Design review of the part built by this model. Coordinates are the model's own, in mm. Face numbers are marked on the shaded views. Give positions to 0.01 mm unless a question says otherwise; leave off trailing zeros. Loops run counter-clockwise (first coordinate to the right, second up) from the corner with the lowest first, then second, coordinate; pieces in that order, holes last. Notation, with made-up numbers: M 34.5,65 L 39.5,65 A8 cw 39.5,77 Z; hole C 78.5,33 d10. An arc over 180 degrees is marked long. Answer as CSV lines item,"result".
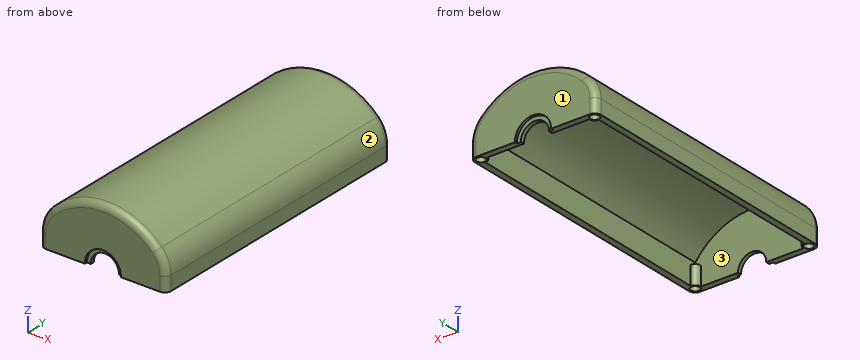
```python
from build123d import *

# Parameters (mm, degrees)
F0_W      = 20
F0_H      = 4
F1_DEPTH  = 45
F2_T      = -1
F3_R      = 5
F4_R      = 5
F6_DEPTH  = 3
F7_R      = 0.7
F8_DEPTH  = 3
F9_R      = 1
F10_R     = 1
F12_DEPTH = 50
F13_DEPTH = 0.4
F15_DEPTH = 0.4


with BuildPart() as f1:
    # F0 (on Front) → F1 (new body)
    with BuildSketch(Plane.XZ):
        with Locations((10, 2)):
            Rectangle(F0_W, F0_H)
        with BuildLine():
            ThreePointArc((20, 4), (10, 9.301808562), (0, 4))
            Line((0, 4), (20, 4))
        make_face()
    extrude(amount=F1_DEPTH)

    # F2
    f2_openings = [f1.faces().sort_by_distance(p)[0] for p in [
        (10, -22.5, 0),
    ]]
    offset(amount=F2_T, openings=f2_openings)

    # F3
    f3_edges = [f1.edges().sort_by_distance(p)[0] for p in [
        (0, -22.5, 4),
    ]]
    fillet(f3_edges, radius=F3_R)

    # F4
    f4_edges = [f1.edges().sort_by_distance(p)[0] for p in [
        (20, -22.5, 4),
    ]]
    fillet(f4_edges, radius=F4_R)

    # F5 (on face) → F6 (join)
    with BuildSketch(Plane(origin=(0, 0, 0), x_dir=(1, 0, 0), z_dir=(0, 0, -1))):
        with BuildLine():
            Line((1, 1), (1.9, 1))
            ThreePointArc((1.9, 1), (1.6363961031, 1.6363961031), (1, 1.9))
            Line((1, 1.9), (1, 1))
        make_face()
        with BuildLine():
            ThreePointArc((19, 1.9), (18.3636038969, 1.6363961031), (18.1, 1))
            Line((18.1, 1), (19, 1))
            Line((19, 1), (19, 1.9))
        make_face()
        with BuildLine():
            ThreePointArc((18.1, 44), (18.3636038969, 43.3636038969), (19, 43.1))
            Line((19, 43.1), (19, 44))
            Line((19, 44), (18.1, 44))
        make_face()
        with BuildLine():
            Line((1, 44), (1, 43.1))
            ThreePointArc((1, 43.1), (1.6363961031, 43.3636038969), (1.9, 44))
            Line((1.9, 44), (1, 44))
        make_face()
    extrude(amount=-F6_DEPTH)

    # F7 (on face) → F8 (cut)
    with BuildSketch(Plane(origin=(0, 0, 0), x_dir=(1, 0, 0), z_dir=(0, 0, -1))):
        with Locations((1, 1)):
            Circle(F7_R)
        with Locations((19, 1)):
            Circle(F7_R)
        with Locations((1, 44)):
            Circle(F7_R)
        with Locations((19, 44)):
            Circle(F7_R)
    extrude(amount=-F8_DEPTH, mode=Mode.SUBTRACT)

    # F9
    f9_edges = [f1.edges().sort_by_distance(p)[0] for p in [
        (20, -45, 1.117556),
        (19.617968, -45, 4.151977),
        (10, -45, 9.301809),
        (0.382032, -45, 4.151977),
        (0, -45, 1.117556),
    ]]
    fillet(f9_edges, radius=F9_R)

    # F10
    f10_edges = [f1.edges().sort_by_distance(p)[0] for p in [
        (0, 0, 1.117556),
        (0.382032, 0, 4.151977),
        (10, 0, 9.301809),
        (19.617968, 0, 4.151977),
        (20, 0, 1.117556),
    ]]
    fillet(f10_edges, radius=F10_R)

    # F11 (on face) → F12 (cut)
    with BuildSketch(Plane.XZ.offset(45)):
        with BuildLine():
            Line((7.7686794017, 0), (12.2313205983, 0))
            ThreePointArc((12.2313205983, 0), (10, 2.2313205983), (7.7686794017, 0))
        make_face()
    extrude(amount=-F12_DEPTH, mode=Mode.SUBTRACT)

    # F11 (on face) → F13 (cut)
    with BuildSketch(Plane.XZ.offset(45)):
        with BuildLine():
            Line((12.2313205983, 0), (12.8707642747, 0))
            ThreePointArc((12.8707642747, 0), (10, 2.8707642747), (7.1292357253, 0))
            Line((7.1292357253, 0), (7.7686794017, 0))
            ThreePointArc((7.7686794017, 0), (10, 2.2313205983), (12.2313205983, 0))
        make_face()
    extrude(amount=-F13_DEPTH, mode=Mode.SUBTRACT)

    # F14 (on face) → F15 (cut)
    with BuildSketch(Plane(origin=(0, 0, 0), x_dir=(-1, 0, 0), z_dir=(0, 1, 0))):
        with BuildLine():
            Line((-7.7686794017, 0), (-7.1292357253, 0))
            ThreePointArc((-7.1292357253, 0), (-10, 2.8707642747), (-12.8707642747, 0))
            Line((-12.8707642747, 0), (-12.2313205983, 0))
            ThreePointArc((-12.2313205983, 0), (-10, 2.2313205983), (-7.7686794017, 0))
        make_face()
    extrude(amount=-F15_DEPTH, mode=Mode.SUBTRACT)


solid = f1.part
```
1. For P1, Ø2, axis at y = -12, z = 5, coming from the -X side; P2, Ø1.3, axis at x = 1, y = -1, coming from the +Z side; P3, Ø3, axis at x = 9, z = 0.5, coming from the +Y side, all flat-tipped, find the tip position at first contact; note any pin that passes through.
Answer block:
P1,"x = 0.32"
P2,"z = 5.95"
P3,"y = -0.4"
2. We need section B-B, the plane y = -23.5. Write out the cut boundary in (x, z).
Answer block:
outline,"M 0,0 L 1,0 L 1,3.69 A11.08 cw 19,3.69 L 19,0 L 20,0 L 20,2.24 A5 ccw 18.53,5.78 A12.08 ccw 1.47,5.78 A5 ccw 0,2.24 Z"
3. We need section C-C, the plane x = 10. Write out the cut boundary in (y, z).
Answer block:
outline,"M -45,2.87 L -44.6,2.87 L -44.6,2.23 L -44,2.23 L -44,8.3 L -1,8.3 L -1,2.23 L -0.4,2.23 L -0.4,2.87 L 0,2.87 L 0,8.3 A1 ccw -1,9.3 L -44,9.3 A1 ccw -45,8.3 Z"
4. We need section A-A, the plane z = 1. Count the separate pieces of the cut face and the enclosed holes in it, plus the area to 3 significant figures.
Answer block:
separate pieces,"2"
enclosed holes,"4"
area,"112 mm²"
5. The part is to be moulded in two halves that separate along Y. For the marked faces 1, 2 and 3, say which applies: pulls with the +Y half, pulls with the -Y half, needs draft (parallel to the pull), parting line crosses it, or undercut.
Answer block:
face 1,"pulls with the +Y half"
face 2,"needs draft"
face 3,"undercut"
6. To check wall thickness, follow L1, parallel to Y at x = 6.25, z = 5.5; L2, parallel to X at y = -22.5, z = 2; L3, parallel to Y at x = 7.25, z = 8. State the ranges of each line that lie inside material, in increasing order. Write a range as [from, to].
Answer block:
L1,"[-45, -44], [-1, 0]"
L2,"[0, 1], [19, 20]"
L3,"[-45, 0]"
